Autodesk Inventor part; units mm, degrees
ref_plane "YZ Plane" through (0, 0, 0) normal (1, 0, 0) x (0, 1, 0)
ref_plane "XZ Plane" through (0, 0, 0) normal (0, 1, 0) x (-1, 0, 0)
ref_plane "XY Plane" through (0, 0, 0) normal (0, 0, 1) x (1, 0, 0)
sketch "Sketch1" plane through (0, 0, 0) normal (0, 0, 1) x (1, 0, 0)
  line L0 (17.5, 11.2702) -> (17.5, 14.0313)
  line L1 (-17.5, 14.0313) -> (-17.5, 11.2702)
  line L2 (20.5, 12.771) -> (20.5, 15.6525)
  line L3 (-20.5, 15.6525) -> (-20.5, 12.771)
  arc A0 (17.5, 14.0313) -> (-17.5, 14.0313) centre (0, 50) ccw
  line L4 (40, 50.029) -> (42.2274, 54.8057)
  line L5 (39.7713, 54.271) -> (41.6722, 58.3474)
  circle A1 centre (0, 50) radius 42.5
  arc A2 (-41.0627, 60.9592) -> (-38.9529, 59.0922) centre (1.7976, 107.2672) ccw
  arc A3 (-18.7749, 88.1281) -> (-16.8719, 86.2676) centre (1.7976, 107.2672) ccw
  arc A4 (-16.8563, 89.0143) -> (-14.8286, 87.1499) centre (1.7976, 107.2672) ccw
  line L6 (16.2129, 86.5669) -> (17.2697, 88.8331)
  line L7 (14.3631, 87.3323) -> (15.422, 89.6032)
  arc A5 (-41.5922, 58.7372) -> (-39.406, 56.8678) centre (1.7976, 107.2672) ccw
  circle A6 centre (0, 55) radius 4
  line L8 (-6, 53.75) -> (6, 53.75)
  line L9 (6, 53.75) -> (6, 56.25)
  line L10 (6, 56.25) -> (-6, 56.25)
  line L11 (-6, 56.25) -> (-6, 53.75)
  point P0 (0, 0)
  point P1 (20.5, 12.771)
  point P2 (42.2274, 54.8057)
  point P3 (-17.5, 11.2702)
  point P4 (17.5, 11.2702)
  point P5 (41.6722, 58.3474)
  point P6 (15.422, 89.6032)
  point P7 (17.2697, 88.8331)
  point P8 (-18.7749, 88.1281)
  point P9 (-16.8563, 89.0143)
  point P10 (-41.0627, 60.9592)
  point P11 (-3.7997, 53.75)
  point P12 (3.7997, 53.75)
  point P13 (3.7997, 56.25)
  point P14 (-3.7997, 56.25)
  point P15 (0, 44.1942)
  dimension "d87" = 40
  dimension "d167" = 85
  dimension "d168" = 2.5
  dimension "d33" = 2
  dimension "d79" = 3
  dimension "d80" = 3
  dimension "d81" = 35
  dimension "d92" = 2
  dimension "d93" = 35
  dimension "d94" = 50
  dimension "d95" = 17.5
  dimension "d146" = 8
  dimension "d147" = 12
  dimension "d148" = 2.5
  dimension "d153" = 55
  dimension "d154" = 1.25
  dimension "d169" = 35
extrude "Extrusion12" add sketch "Sketch1" along normal blind 5 contours A1 L1 A0 L0 | L0 A0 L2 A1 | A1 L3 A0 L1 | L2 A0 L4 A1 | A1 A5 A0 L3 | A0 L5 A1 L4 | A1 A2 A0 A5 | A0 L6 A1 L5 | A1 A3 A0 A2 | A0 L7 A1 L6 | A1 A4 A0 A3 | A0 A4 A1 L7 | A6 L8 L10 | A6 L10 L9 L8 | L10 A6 | A6 L8 | A6 L8 L11 L10
extrude "Extrusion13" add sketch "Sketch1" along normal blind 5 contours A1 L1 A0 L0 | A6 L8 L10 | A6 L10 L9 L8 | L10 A6 | A6 L8 | A6 L8 L11 L10
extrude "Extrusion14" cut sketch "Sketch1" along normal blind 17 contours A6 L8 L10 | A6 L10 L9 L8 | L10 A6 | A6 L8 | A6 L8 L11 L10
extrude "Extrusion15" add sketch "Sketch1" along normal blind 5 contours A6 L10 L9 L8 | A6 L8 L11 L10
extrude "Extrusion16" add sketch "Sketch1" along normal blind 30 contours L2 A0 L4 A1 | A1 A5 A0 L3 | A0 L7 A1 L6 | A0 A4 A1 L7
extrude "Extrusion17" add sketch "Sketch1" along normal blind 30 contours L0 A0 L2 A1 | A1 L3 A0 L1 | A0 L5 A1 L4 | A1 A2 A0 A5 | A1 A4 A0 A3
extrude "Extrusion18" cut sketch "Sketch1" along normal blind 30 contours L0 A0 L2 A1 | A1 L3 A0 L1 | A0 L5 A1 L4 | A1 A2 A0 A5 | A0 L7 A1 L6 | A1 A4 A0 A3
extrude "Extrusion19" add sketch "Sketch1" along normal blind 5 contours L0 A0 L2 A1 | A1 L3 A0 L1 | A0 L5 A1 L4 | A1 A2 A0 A5 | A0 L7 A1 L6 | A1 A4 A0 A3
Geometry: final body of the model. Coordinates: model frame, mm. A direction names the side the tool comes from. Coordinates: 2 decimals unless noted, no trailing zeros. Loops run counter-clockwise (first coordinate to the right, second up) from the corner with the lowest first, then second, coordinate; pieces in that order, holes last. Notation, with made-up numbers: (-30.5, -37.5) -> (5.5, -37.5) arc R28 ccw to (5.5, -17.5) -> close; hole circle Ø1 at (66.5, -38.75). An arc over 180 degrees is marked (long way). Use a Markdown table: item, result. Add a question column.
(1) Section query A-A, the plane x = 0. Return loops of the section in (y, z).
(2) Section query D-D, the plane x = 11. Return loops of the section in (y, z), plus the area to 3 significant figures.
(3) Section query C-C, the plane z = 14. Return loops of the section in (x, y).
(4) Section query B-B, the plane y = 43. Return loops of the section in (x, z), plus the area to 3 significant figures.
(5) Pin query (flat end, axial travel): pin 1 Ø3 at (y, z) = (57.5, 20.5) entering from +X; pin 2 Ø0.9 at (y, z) = (13.5, 22) entering from +X; pin 3 Ø0.9 at (y, z) = (14, 22.5) entering from -X. Return the tip coordinate at first contact, or that it passes through.
(6) Access query for faces 1 (the flat face through (-20.5, 14, 17)), 2 (the flat face through (41.098, 52.384, 17.325)), 3 (the cylindrical face through (0, 90, 17)), 4 (the cylindrical face through (-36.215, 33.016, 17.325)). Directions: +Z, -Z, +X, -X, +Y, -Y. A direction counts if a zero-diameter tool reaches every point of the face in a straight line with its end or side. Return the directions, or none.
(7) Mould query, pull axis Y, two halves, no side actions, for faces 5 (the flat face through (-0.6, 50.6, 0)), 6 (the flat face through (14.885, 88.452, 17.325)), 7 (the cylindrical face through (3.03, 57.61, 2.46)). Classes: pulls with the +Y half, pulls with the -Y half, needs draft (parallel to the pull), parting line crosses it, or undercut.
(8) Line query: line 1 along Y through (x, z) = (0, 2.95); line 2 along Z through (x, y) = (-19.5, 83); line 3 along X through (y, z) = (55, 3.55). Output: solid intervals per line, ascending.
Answer:
| question | item | result |
|---|---|---|
| 1 | outline | (7.5, 0) -> (51, 0) -> (51, 5) -> (7.5, 5) -> close; (59, 0) -> (92.5, 0) -> (92.5, 30) -> (90, 30) -> (90, 5) -> (59, 5) -> close |
| 2 | outline | (8.95, 0) -> (91.05, 0) -> (91.05, 30) -> (88.46, 30) -> (88.46, 5) -> (8.95, 5) -> close |
| 2 | area | 475 mm^2 |
| 3 | outline | (-41.59, 58.74) arc R42.5 ccw to (-20.5, 12.77) -> (-20.5, 15.65) arc R40 cw to (-39.41, 56.87) arc R65.11 cw to start; (-16.86, 89.01) arc R26.1 ccw to (-14.83, 87.15) arc R40 cw to (14.36, 87.33) -> (15.42, 89.6) arc R42.5 ccw to start; (20.5, 12.77) arc R42.5 ccw to (42.23, 54.81) -> (40, 50.03) arc R40 cw to (20.5, 15.65) -> close |
| 4 | outline | (-41.92, 0) -> (41.92, 0) -> (41.92, 30) -> (39.38, 30) -> (39.38, 5) -> (-39.38, 5) -> (-39.38, 30) -> (-41.92, 30) -> close |
| 4 | area | 546 mm^2 |
| 5 | pin 1 | stops at x = -39.41 |
| 5 | pin 2 | stops at x = 22.51 |
| 5 | pin 3 | stops at x = -23.29 |
| 6 | face 1 | +Z, +Y, -Y |
| 6 | face 2 | +Z, +Y |
| 6 | face 3 | +Z, -Y |
| 6 | face 4 | +Z |
| 7 | face 5 | needs draft |
| 7 | face 6 | pulls with the -Y half |
| 7 | face 7 | undercut |
| 8 | line 1 | y = 7.5 to 51, 59 to 92.5 |
| 8 | line 2 | z = 0 to 5 |
| 8 | line 3 | x = -42.2 to -4, 4 to 42.2 |
